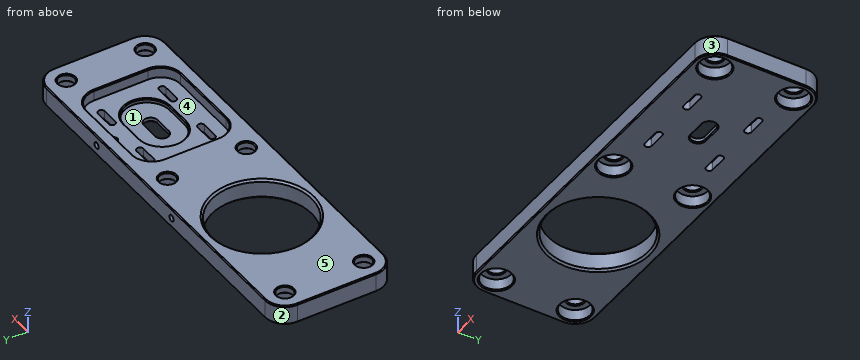
```python
from build123d import *

# Parameters (mm, degrees)
SKICA1_W                  = 195
SKICA1_H                  = 60
P_IDAT_VYSUNUT_M1_DEPTH   = 10
ODEBRAT_VYSUNUT_M1_DEPTH  = 10
ODEBRAT_VYSUNUT_M3_DEPTH  = 2
SKICA6_R                  = 25.25
ODEBRAT_VYSUNUT_M5_DEPTH  = 10
SKICA8_W                  = 56.5
SKICA8_H                  = 47.5
ODEBRAT_VYSUNUT_M7_DEPTH  = 5.57
ODEBRAT_VYSUNUT_M8_DEPTH  = 2.1
ZKOSEN_2_SIZE             = 1
ZKOSEN_4_SIZE             = 0.5
ZAOBLIT2_R                = 10
SKICA12_R                 = 4.1
ODEBRAT_VYSUNUT_M10_DEPTH = 10
SKICA13_R                 = 7.5
ODEBRAT_VYSUNUT_M11_DEPTH = 6
ZKOSEN_6_SIZE             = 0.5
ZAOBLIT4_R                = 10
ZKOSEN_7_SIZE             = 0.5
ZKOSEN_8_SIZE             = 0.5
M4_Z_VIT2_D               = 3.3
M4_Z_VIT2_DEPTH           = 10
M4_Z_VIT2_TIP             = 0.991420021


with BuildPart() as part:
    # Skica1 → Přidat vysunutím1 (new body)
    with BuildSketch(Plane.XY):
        with Locations((97.5, 30)):
            Rectangle(SKICA1_W, SKICA1_H)
    extrude(amount=P_IDAT_VYSUNUT_M1_DEPTH)

    # Skica2 → Odebrat vysunutím1 (cut)
    with BuildSketch(Plane.XY.offset(10)):
        with BuildLine():
            Line((133.1, 43.8), (124.5, 43.8))
            ThreePointArc((124.5, 43.8), (122.8, 45.5), (124.5, 47.2))
            Line((124.5, 47.2), (133.1, 47.2))
            ThreePointArc((133.1, 47.2), (134.8, 45.5), (133.1, 43.8))
        make_face()
        with BuildLine():
            Line((164.1, 43.8), (155.5, 43.8))
            ThreePointArc((155.5, 43.8), (153.8, 45.5), (155.5, 47.2))
            Line((155.5, 47.2), (164.1, 47.2))
            ThreePointArc((164.1, 47.2), (165.8, 45.5), (164.1, 43.8))
        make_face()
        with BuildLine():
            Line((133.1, 16.2), (124.5, 16.2))
            ThreePointArc((124.5, 16.2), (122.8, 14.5), (124.5, 12.8))
            Line((124.5, 12.8), (133.1, 12.8))
            ThreePointArc((133.1, 12.8), (134.8, 14.5), (133.1, 16.2))
        make_face()
        with BuildLine():
            Line((164.1, 16.2), (155.5, 16.2))
            ThreePointArc((155.5, 16.2), (153.8, 14.5), (155.5, 12.8))
            Line((155.5, 12.8), (164.1, 12.8))
            ThreePointArc((164.1, 12.8), (165.8, 14.5), (164.1, 16.2))
        make_face()
        with BuildLine():
            Line((149, 26.5), (140, 26.5))
            ThreePointArc((140, 26.5), (136.5, 30), (140, 33.5))
            Line((140, 33.5), (149, 33.5))
            ThreePointArc((149, 33.5), (152.5, 30), (149, 26.5))
        make_face()
    extrude(amount=-ODEBRAT_VYSUNUT_M1_DEPTH, mode=Mode.SUBTRACT)

    # Skica5 → Odebrat vysunutím3 (cut)
    with BuildSketch(Plane.XY.offset(10)):
        with BuildLine():
            Line((148, 19), (140, 19))
            ThreePointArc((140, 19), (129, 30), (140, 41))
            Line((140, 41), (148, 41))
            ThreePointArc((148, 41), (159, 30), (148, 19))
        make_face()
    extrude(amount=-ODEBRAT_VYSUNUT_M3_DEPTH, mode=Mode.SUBTRACT)

    # Skica6 → Odebrat vysunutím5 (cut)
    with BuildSketch(Plane(origin=(0, 0, 0), x_dir=(-1, 0, 0), z_dir=(0, 0, -1))):
        with Locations((-60, 30)):
            Circle(SKICA6_R)
    extrude(amount=-ODEBRAT_VYSUNUT_M5_DEPTH, mode=Mode.SUBTRACT)

    # Skica8 → Odebrat vysunutím7 (cut)
    with BuildSketch(Plane.XY.offset(10)):
        with Locations((144.5, 30)):
            Rectangle(SKICA8_W, SKICA8_H)
    extrude(amount=-ODEBRAT_VYSUNUT_M7_DEPTH, mode=Mode.SUBTRACT)

    # Skica9 → Odebrat vysunutím8 (cut)
    with BuildSketch(Plane.XY.offset(4.43)):
        with BuildLine():
            Line((152, 18.5), (140, 18.5))
            ThreePointArc((140, 18.5), (128.5, 30), (140, 41.5))
            Line((140, 41.5), (152, 41.5))
            ThreePointArc((152, 41.5), (163.5, 30), (152, 18.5))
        make_face()
    extrude(amount=-ODEBRAT_VYSUNUT_M8_DEPTH, mode=Mode.SUBTRACT)

    # Zkosení2
    zkosen_2_edges = [part.edges().sort_by_distance(p)[0] for p in [
        (85.25, 30, 0),
        (85.25, 30, 10),
    ]]
    chamfer(zkosen_2_edges, length=ZKOSEN_2_SIZE)

    # Zkosení4
    zkosen_4_edges = [part.edges().sort_by_distance(p)[0] for p in [
        (144.5, 33.5, 0),
        (136.5, 30, 0),
        (144.5, 26.5, 0),
        (152.5, 30, 0),
    ]]
    chamfer(zkosen_4_edges, length=ZKOSEN_4_SIZE)

    # Zaoblit2
    zaoblit2_edges = [part.edges().sort_by_distance(p)[0] for p in [
        (0, 60, 5),
        (195, 60, 5),
        (195, 0, 5),
        (0, 0, 5),
    ]]
    fillet(zaoblit2_edges, radius=ZAOBLIT2_R)

    # Skica12 → Odebrat vysunutím10 (cut)
    with BuildSketch(Plane(origin=(0, 0, 0), x_dir=(-1, 0, 0), z_dir=(0, 0, -1))):
        with Locations((-10, 50)):
            Circle(SKICA12_R)
        with Locations((-10, 10)):
            Circle(SKICA12_R)
        with Locations((-104, 50)):
            Circle(SKICA12_R)
        with Locations((-104, 10)):
            Circle(SKICA12_R)
        with Locations((-185, 50)):
            Circle(SKICA12_R)
        with Locations((-185, 10)):
            Circle(SKICA12_R)
    extrude(amount=-ODEBRAT_VYSUNUT_M10_DEPTH, mode=Mode.SUBTRACT)

    # Skica13 → Odebrat vysunutím11 (cut)
    with BuildSketch(Plane(origin=(0, 0, 0), x_dir=(-1, 0, 0), z_dir=(0, 0, -1))):
        with Locations((-10, 50)):
            Circle(SKICA13_R)
        with Locations((-10, 10)):
            Circle(SKICA13_R)
        with Locations((-104, 50)):
            Circle(SKICA13_R)
        with Locations((-104, 10)):
            Circle(SKICA13_R)
        with Locations((-185, 50)):
            Circle(SKICA13_R)
        with Locations((-185, 10)):
            Circle(SKICA13_R)
    extrude(amount=-ODEBRAT_VYSUNUT_M11_DEPTH, mode=Mode.SUBTRACT)

    # Zkosení6
    zkosen_6_edges = [part.edges().sort_by_distance(p)[0] for p in [
        (189.1, 50, 10),
        (108.1, 10, 10),
        (108.1, 50, 10),
        (14.1, 10, 10),
        (189.1, 10, 10),
        (14.1, 50, 10),
        (192.5, 50, 0),
        (189.1, 50, 6),
        (111.5, 10, 0),
        (108.1, 10, 6),
        (111.5, 50, 0),
        (108.1, 50, 6),
        (17.5, 10, 0),
        (14.1, 10, 6),
        (192.5, 10, 0),
        (189.1, 10, 6),
        (17.5, 50, 0),
        (14.1, 50, 6),
    ]]
    chamfer(zkosen_6_edges, length=ZKOSEN_6_SIZE)

    # Zaoblit4
    zaoblit4_edges = [part.edges().sort_by_distance(p)[0] for p in [
        (116.25, 6.25, 7.215),
        (116.25, 53.75, 7.215),
        (172.75, 53.75, 7.215),
        (172.75, 6.25, 7.215),
    ]]
    fillet(zaoblit4_edges, radius=ZAOBLIT4_R)

    # Zkosení7
    zkosen_7_edges = [part.edges().sort_by_distance(p)[0] for p in [
        (195, 30, 0),
        (195, 30, 10),
        (0, 30, 0),
        (97.5, 60, 0),
        (97.5, 0, 0),
        (2.928932188, 57.071067812, 0),
        (2.928932188, 2.928932188, 0),
        (192.071067812, 57.071067812, 0),
        (192.071067812, 2.928932188, 0),
        (97.5, 0, 10),
        (0, 30, 10),
        (97.5, 60, 10),
        (2.928932188, 57.071067812, 10),
        (2.928932188, 2.928932188, 10),
        (192.071067812, 57.071067812, 10),
        (192.071067812, 2.928932188, 10),
    ]]
    chamfer(zkosen_7_edges, length=ZKOSEN_7_SIZE)

    # Zkosení8
    zkosen_8_edges = [part.edges().sort_by_distance(p)[0] for p in [
        (163.5, 30, 4.43),
        (146, 41.5, 4.43),
        (128.5, 30, 4.43),
        (146, 18.5, 4.43),
        (144.5, 6.25, 10),
        (116.25, 30, 10),
        (172.75, 30, 10),
        (144.5, 53.75, 10),
        (119.178932188, 9.178932188, 10),
        (169.821067812, 9.178932188, 10),
        (169.821067812, 50.821067812, 10),
        (119.178932188, 50.821067812, 10),
    ]]
    chamfer(zkosen_8_edges, length=ZKOSEN_8_SIZE)

    # M4 závit2
    with Locations(Plane(origin=(0, 60, 0), x_dir=(1, 0, 0), z_dir=(0, 1, 0))):
        with Locations((85, -5), (145, -5)):
            Hole(M4_Z_VIT2_D / 2, depth=M4_Z_VIT2_DEPTH)
            with Locations((0, 0, -(M4_Z_VIT2_DEPTH + M4_Z_VIT2_TIP / 2))):  # 118° drill point
                Cone(0, M4_Z_VIT2_D / 2, M4_Z_VIT2_TIP, mode=Mode.SUBTRACT)


solid = part.part
```
Check sheet for the modelled part. Datum: model origin and axes. Units: mm. Face numbers are marked on the shaded views. A direction names the side the tool comes from. Round coordinates to 2 decimals unless told otherwise and drop trailing zeros. Order: outer loops, then holes, each group sorted by start corner. A loop starts at its lowest first (then second) coordinate and runs counter-clockwise, first axis right, second up. Notation, with made-up numbers: (81, 15) -> (106, 15) arc R20 ccw to (106, 29) -> close; hole circle Ø3 at (-5, 63). An arc over 180 degrees is marked (long way). One line per item, written item: value. Start each with the question number.
Q1. Cross-section at B-B (y = 30). Give the number of separate pieces and of enclosed holes in the cut face, and give its area (3 significant figures).
Q2. Set-up check for the marked faces 1 and 2: record each of +Z, -Z, +X, -X, +Y, -Y from which the full face is reachable in a straight line by a thin tool's end or side.
Q3. Cross-section at A-A (x = 60). Record the boundary of the cut face in (y, z), and give its area (3 significant figures).
Q4. Thickness scan on line 1 (Y direction, x = 10, z = 2.95); line 2 (Y direction, x = 104, z = 8.25); line 3 (X direction, y = 16, z = 9.25). Record the ranges inside material, lowest first.
Q5. Mould release check, pull along X, two halves, no side actions. Record for the marked faces 3, 4 and 5: pulls with the +X half, pulls with the -X half, needs draft (parallel to the pull), parting line crosses it, or undercut.
Q6. Gauge pin test, flat ends, axial feed: pin 1 Ø5 at (x, y) = (10, 50) entering from -Z; pin 2 Ø13.5 at (x, y) = (185, 50) entering from -Z; pin 3 Ø18.5 at (x, y) = (139, 30) entering from +Z; pin 4 Ø7.5 at (x, y) = (13, 12.5) entering from -Z. Record the tip position at first contact, or that the pin passes through.
Completed:
1. separate pieces: 3
1. enclosed holes: 0
1. area: 1,020 mm²
2. face 1: +Z
2. face 2: +Z, -Z, -X, +Y
3. outline: (0, 0.5) -> (0.5, 0) -> (3.75, 0) -> (4.75, 1) -> (4.75, 9) -> (3.75, 10) -> (0.5, 10) -> (0, 9.5) -> close; (55.25, 1) -> (56.25, 0) -> (59.5, 0) -> (60, 0.5) -> (60, 9.5) -> (59.5, 10) -> (56.25, 10) -> (55.25, 9) -> close
3. area: 92.5 mm²
4. line 1: y = 0 to 2.5, 17.5 to 42.5, 57.5 to 60
4. line 2: y = 0 to 5.9, 14.1 to 45.9, 54.1 to 60
4. line 3: x = 0 to 38.69, 81.31 to 116.25, 172.75 to 195
5. face 3: pulls with the +X half
5. face 4: undercut
5. face 5: needs draft
6. pin 1: passes through
6. pin 2: stops at z = 6
6. pin 3: stops at z = 2.33
6. pin 4: stops at z = 0.34
